```python
from build123d import *

# Parameters (mm, degrees)
SKETCH_1_W          = 10
SKETCH_1_H          = 10
SKETCH_1_W_2        = 8
SKETCH_1_H_2        = 8
EXTRUDE_1_DEPTH     = 219
SKETCH_2_R          = 1.5
CUT_EXTRUDE_1_DEPTH = 10
SKETCH_3_R          = 1.5
CUT_EXTRUDE_2_DEPTH = 11


with BuildPart() as part:
    # 草图1 → 拉伸-薄壁1 (new body)
    with BuildSketch(Plane.XY):
        Rectangle(SKETCH_1_W, SKETCH_1_H)
        Rectangle(SKETCH_1_W_2, SKETCH_1_H_2, mode=Mode.SUBTRACT)
    extrude(amount=EXTRUDE_1_DEPTH)

    # 草图2 → 切除-拉伸1 (cut)
    with BuildSketch(Plane(origin=(0, 5, 0), x_dir=(1, 0, 0), z_dir=(0, 1, 0))):
        with Locations((0, -182)):
            Circle(SKETCH_2_R)
        with Locations((0, -20)):
            Circle(SKETCH_2_R)
        with Locations((0, -120)):
            Circle(SKETCH_2_R)
        with Locations((0, -162)):
            Circle(SKETCH_2_R)
        with Locations((0, -75)):
            Circle(SKETCH_2_R)
    extrude(amount=-CUT_EXTRUDE_1_DEPTH, mode=Mode.SUBTRACT)

    # 草图3 → 切除-拉伸2 (cut, through all)
    with BuildSketch(Plane(origin=(5, 0, 0), x_dir=(0, 0, -1), z_dir=(1, 0, 0))):
        with Locations((-13, 0)):
            Circle(SKETCH_3_R)
        with Locations((-28, 0)):
            Circle(SKETCH_3_R)
        with Locations((-138.5, 0)):
            Circle(SKETCH_3_R)
        with Locations((-100, 0)):
            Circle(SKETCH_3_R)
        with Locations((-110, 0)):
            Circle(SKETCH_3_R)
    extrude(amount=-CUT_EXTRUDE_2_DEPTH, mode=Mode.SUBTRACT)


solid = part.part
```
Work out the finished part from the listing and answer in its coordinate system (mm). A direction names the side the tool comes from. Round coordinates to 2 decimals unless told otherwise and drop trailing zeros. Order: outer loops, then holes, each group sorted by start corner. A loop starts at its lowest first (then second) coordinate and runs counter-clockwise, first axis right, second up.
Q1. A cutting plane is placed at A-A, the plane z = 204. Determine the outline of the cut face in (x, y), then the cut area to 3 significant figures.
Solution:
outline: (-5, -5) - (5, -5) - (5, 5) - (-5, 5) - close; hole (-4, -4) - (4, -4) - (4, 4) - (-4, 4) - close
area: 36.0 mm2
Q2. Find the intervals of material crossed by line 1 along Z through (x, y) = (0, -4.4); line 2 along X through (y, z) = (-1, 147); line 3 along X through (y, z) = (-4.2, 75), in increasing order.
Solution:
line 1: z = 0 to 18.5, 21.5 to 73.5, 76.5 to 118.5, 121.5 to 160.5, 163.5 to 180.5, 183.5 to 219
line 2: x = -5 to -4, 4 to 5
line 3: x = -5 to -1.5, 1.5 to 5
Q3. The mould has two halves that part along X. Classify faces 3 (the flat face through (-4, 0, 108)), 4 (the flat face through (-5, 0, 108)), 5 (the flat face through (-4.5, 0.1, 219)): pulls with the +X half, pulls with the -X half, needs draft (parallel to the pull), parting line crosses it, or undercut.
Solution:
face 3: undercut
face 4: pulls with the -X half
face 5: needs draft
Q4. Given pin 1 Ø2.5 at (x, z) = (0, 20) entering from +Y, flat-ended and moving along its own axis, determine where the tip first touches the part or whether it passes through.
Solution:
pin 1: passes through
Q5. A tool of negligible diameter and unlimited length cuts with its end or side. For faces 1 (the flat face through (0, -4, 108)), 2 (the flat face through (-4.5, 0.1, 0)), from which of +Z, -Z, +X, -X, +Y, -Y can it reach the whole face along a straight path? Write none if from no direction.
Solution:
face 1: +Z, -Z
face 2: -Z, +X, -X, +Y, -Y
